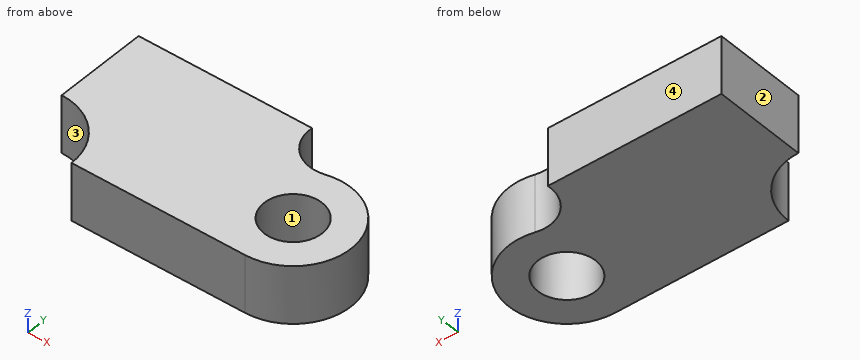
from build123d import *

# Parameters (mm, degrees)
F0_R     = 5
F1_DEPTH = 10


with BuildPart() as f1:
    # F0 (on Top) → F1 (new body)
    with BuildSketch(Plane.XY):
        with BuildLine():
            Line((-30, -10), (-10, -10))
            Line((-10, -10), (0, -10))
            ThreePointArc((0, -10), (9.919398, 1.2671), (-2.513773, 9.678892))
            ThreePointArc((-2.513773, 9.678892), (-7.89291, 10.901868), (-10, 16))
            Line((-10, 16), (-40, 16))
            Line((-40, 16), (-40, 0))
            ThreePointArc((-40, 0), (-32.928932, -2.928932), (-30, -10))
        make_face()
        Circle(F0_R, mode=Mode.SUBTRACT)
    extrude(amount=F1_DEPTH)


solid = f1.part
The model under review builds one solid part; all positions refer to its coordinate system, in mm. Face numbers are marked on the shaded views. Give positions to 0.01 mm unless a question says otherwise; leave off trailing zeros. Write each loop counter-clockwise with the first axis right and the second up, starting at its lowest first coordinate (ties: lowest second). Pieces come first, ordered by that corner, then holes.
1. For P1, Ø5, axis at x = 0.5, z = 6.5, coming from the +Y side, flat-tipped, find the tip position at first contact; note if it passes through.
2. Draft analysis for pull direction Y (two halves, no side actions). For the marked faces 1, 2, 3 and 4, state which applies: +Y half, -Y half, draft (parallel to the pull), parting line (faces both ways), or undercut.
3. Add section A-A, the plane y = -1. Write out the cut boundary in (x, z).
4. Add section B-B, the plane z = 6.75. Write out the cut boundary in (x, y), plus the area to 3 significant figures.
5. Add section C-C, the plane x = -35.5. Write out the cut boundary in (y, z).
6. Add section D-D, the plane y = 13.5. Write out the cut boundary in (x, z), plus the area to 3 significant figures.
7. Wall thickness on L1, parallel to Y at x = 0, z = 6.5; L2, parallel to X at y = 15, z = 5; L3, parallel to Y at x = -4, z = 2: over which ranges is each line inside the solid? List them lowest first.
Worked answers:
1. P1: stops at y = 10
2. face 1: undercut
2. face 2: draft
2. face 3: -Y half
2. face 4: +Y half
3. outline: (-35.64, 0) - (-4.9, 0) - (-4.9, 10) - (-35.64, 10) - close; (4.9, 0) - (9.95, 0) - (9.95, 10) - (4.9, 10) - close
4. outline: (-40, 0) arc R10 cw to (-30, -10) - (0, -10) arc R10 ccw (long way) to (-2.51, 9.68) arc R6 cw to (-10, 16) - (-40, 16) - close; hole circle Ø10 at (0, 0)
4. area: 984 mm2
5. outline: (-1.07, 0) - (16, 0) - (16, 10) - (-1.07, 10) - close
6. outline: (-40, 0) - (-9.68, 0) - (-9.68, 10) - (-40, 10) - close
6. area: 303 mm2
7. L1: y = -10 to -5, 5 to 10
7. L2: x = -40 to -10
7. L3: y = -10 to -3, 3 to 9.49
